from build123d import *

# Parameters (mm, degrees)
SKETCH1_R                       = 10
BOSS_EXTRUDE1_DEPTH             = 0.1
BOSS_EXTRUDE2_START             = -2.28
SKETCH3_W                       = 4.5
SKETCH3_H                       = 2.5
BOSS_EXTRUDE2_DEPTH             = 0.1
EXTRUDE_THIN1_REACH             = 17.432
EXTRUDE_THIN1_DIRECTION_2_REACH = 17.432


with BuildPart() as part:
    # Sketch1 → Boss-Extrude1 (new body)
    with BuildSketch(Plane(origin=(0, 1.1, 0), x_dir=(1, 0, 0), z_dir=(0, 1, 0))):
        with Locations(Location((0, 1.53064501, 0), (0, 0, 270))):
            Circle(SKETCH1_R)
    extrude(amount=BOSS_EXTRUDE1_DEPTH)


with BuildPart() as body_2:
    # Sketch3 → Boss-Extrude2 (new body)
    with BuildSketch(Plane(origin=(0, 0, 0), x_dir=(1, 0, 0), z_dir=(0, 1, 0)).offset(BOSS_EXTRUDE2_START)):
        with Locations((0, -9.25)):
            Rectangle(SKETCH3_W, SKETCH3_H)
    extrude(amount=BOSS_EXTRUDE2_DEPTH)

    # Extrude-Thin1: up to this face of the body (flat: up to its plane)
    extrude_thin1_end = Plane(body_2.part.faces().sort_by_distance((2.25, -2.23, 9.25))[0])
    # Sketch4 → Extrude-Thin1 (add, up to the picked face)
    with BuildSketch(Plane(origin=(0, 0, 0), x_dir=(0, 0, -1), z_dir=(1, 0, 0)), mode=Mode.PRIVATE) as extrude_thin1_sk1:
        with BuildLine():
            Line((-9.5, -2.28), (-10.5, -2.28))
            Line((-10.5, -2.28), (-11, -2.28))
            ThreePointArc((-11, -2.28), (-11.452530048, -2.113120853), (-11.688368572, -1.692392575))
            ThreePointArc((-11.688368572, -1.692392575), (-11.120799367, 0.32311715), (-9.21935499, 1.2))
            Line((-9.21935499, 1.2), (-8.46935499, 1.2))
            Line((-8.46935499, 1.2), (-5, 1.2))
            Line((-5, 1.2), (-5, 1.1))
            Line((-5, 1.1), (-8.46935499, 1.1))
            Line((-8.46935499, 1.1), (-9.21935499, 1.1))
            ThreePointArc((-9.21935499, 1.1), (-11.044741592, 0.258192464), (-11.589608029, -1.676696872))
            ThreePointArc((-11.589608029, -1.676696872), (-11.387605362, -2.037063078), (-11, -2.18))
            Line((-11, -2.18), (-10.5, -2.18))
            Line((-10.5, -2.18), (-9.5, -2.18))
            Line((-9.5, -2.18), (-9.5, -2.28))
        make_face()
    extrude_thin1_tool1 = split(extrude(extrude_thin1_sk1.sketch, amount=EXTRUDE_THIN1_REACH, mode=Mode.PRIVATE), bisect_by=extrude_thin1_end, keep=Keep.BOTH, mode=Mode.PRIVATE)

    add(part.part)  # Extrude-Thin1 merges part
    add(extrude_thin1_tool1.solids().sort_by(Axis((0, -2.25567, 10.75), (1, 0, 0)))[0])

    # Extrude-Thin1 direction 2: up to this face of the body (flat: up to its plane)
    extrude_thin1_direction_2_end = Plane(body_2.part.faces().sort_by_distance((-2.25, -2.23, 9.25))[0])
    # Sketch4 → Extrude-Thin1 direction 2 (add, up to the picked face)
    with BuildSketch(Plane(origin=(0, 0, 0), x_dir=(0, 0, -1), z_dir=(1, 0, 0)), mode=Mode.PRIVATE) as extrude_thin1_direction_2_sk1:
        with BuildLine():
            Line((-9.5, -2.28), (-10.5, -2.28))
            Line((-10.5, -2.28), (-11, -2.28))
            ThreePointArc((-11, -2.28), (-11.452530048, -2.113120853), (-11.688368572, -1.692392575))
            ThreePointArc((-11.688368572, -1.692392575), (-11.120799367, 0.32311715), (-9.21935499, 1.2))
            Line((-9.21935499, 1.2), (-8.46935499, 1.2))
            Line((-8.46935499, 1.2), (-5, 1.2))
            Line((-5, 1.2), (-5, 1.1))
            Line((-5, 1.1), (-8.46935499, 1.1))
            Line((-8.46935499, 1.1), (-9.21935499, 1.1))
            ThreePointArc((-9.21935499, 1.1), (-11.044741592, 0.258192464), (-11.589608029, -1.676696872))
            ThreePointArc((-11.589608029, -1.676696872), (-11.387605362, -2.037063078), (-11, -2.18))
            Line((-11, -2.18), (-10.5, -2.18))
            Line((-10.5, -2.18), (-9.5, -2.18))
            Line((-9.5, -2.18), (-9.5, -2.28))
        make_face()
    extrude_thin1_direction_2_tool1 = split(extrude(extrude_thin1_direction_2_sk1.sketch, amount=-EXTRUDE_THIN1_DIRECTION_2_REACH, mode=Mode.PRIVATE), bisect_by=extrude_thin1_direction_2_end, keep=Keep.BOTH, mode=Mode.PRIVATE)
    add(extrude_thin1_direction_2_tool1.solids().sort_by(Axis((0, -2.25567, 10.75), (-1, 0, 0)))[0])


solid = body_2.part
Input: part model. Units: mm. Frame: model coordinates. Coordinates: 2 decimals unless noted, no trailing zeros. Order: outer loops, then holes, each group sorted by start corner. A loop starts at its lowest first (then second) coordinate and runs counter-clockwise, first axis right, second up. Notation, with made-up numbers: M 67,77.25 L 101,77.25 A21 ccw 101,114.25 Z; hole C 32,3 d8. An arc over 180 degrees is marked long. Answer as CSV lines item,"result".
1. First-contact query: P1, Ø12, axis at x = 3.5, z = -2.5, coming from the -Y side. Flat tip, straight axial feed; report the tip coordinate or a pass-through.
Reported:
P1,"y = 1.1"
2. Section B-B (y = -0.45). Return the cut outline in (x, z), then the cut area to 3 significant figures.
Reported:
outline,"M -2.25,11.46 L 2.25,11.46 L 2.25,11.57 L -2.25,11.57 Z"
area,"0.480 mm2"
3. Material intervals for line 1 (Z direction, x = 1.5, y = 0.9), sorted ascending. Write a range as from..to.
Reported:
line 1,"10.18..10.41"
4. Section C-C (z = -7.25). Return the cut outline in (x, y), then the cut area to 3 significant figures.
Reported:
outline,"M -8.2,1.1 L 8.2,1.1 L 8.2,1.2 L -8.2,1.2 Z"
area,"1.64 mm2"
5. Section A-A (x = 0). Return the cut outline in (y, z), then the cut area to 3 significant figures.
Reported:
outline,"M -2.28,8 L -2.18,8 L -2.18,11 A0.6 cw -1.68,11.59 A2.4 cw 1.1,9.22 L 1.1,-11.53 L 1.2,-11.53 L 1.2,9.22 A2.5 ccw -1.69,11.69 A0.7 ccw -2.28,11 Z"
area,"2.89 mm2"
